Geometry check sheet. Reference: the model listing, model coordinates, mm. A direction names the side the tool comes from. Round coordinates to 2 decimals unless told otherwise and drop trailing zeros. Write each loop counter-clockwise with the first axis right and the second up, starting at its lowest first coordinate (ties: lowest second). Pieces come first, ordered by that corner, then holes. Notation, with made-up numbers: (18.5, 43) - (71.5, 43) arc R25 ccw to (71.5, 75) - close; hole circle Ø6 at (80.5, -34.5). An arc over 180 degrees is marked (long way). Return JSON: item names as keys, results as strings. Group by question number.
from build123d import *

# Parameters (mm, degrees)
SKETCH1_R               = 140
BOSS_EXTRUDE1_DEPTH     = 4
CUT_EXTRUDE1_REACH      = 6
CUT_EXTRUDE3_REACH      = 6
SKETCH19_R              = 1.5
CUT_EXTRUDE4_REACH      = 6
FILLET2_R               = 10
CUT_EXTRUDE8_DEPTH      = 1
CUT_EXTRUDE8_DEPTH_BACK = 5
CUT_EXTRUDE9_REACH      = 6
FILLET4_R               = 5
FILLET6_R               = 10
CUT_EXTRUDE10_REACH     = 6
SKETCH25_R              = 1.5
FILLET5_R               = 3


with BuildPart() as part:
    # Sketch1 → Boss-Extrude1 (new body)
    with BuildSketch(Plane(origin=(0, 0, 0), x_dir=(1, 0, 0), z_dir=(0, 1, 0))):
        Circle(SKETCH1_R)
    extrude(amount=BOSS_EXTRUDE1_DEPTH)

    # Sketch17 → Cut-Extrude1 (cut, up to next)
    with BuildSketch(Plane.XZ, mode=Mode.PRIVATE) as cut_extrude1_sk1:
        Polygon((-50, 90), (-121.24355653, 70), (-121.24355653, 140), (121.24355653, 140), (121.24355653, 70), (50, 90), align=None)
    cut_extrude1_tool1 = extrude(cut_extrude1_sk1.sketch, amount=-CUT_EXTRUDE1_REACH, mode=Mode.PRIVATE) & part.part
    add(cut_extrude1_tool1.solids().sort_by_distance((0, 0, 111.669853))[0], mode=Mode.SUBTRACT)

    # Sketch19 → Cut-Extrude3 (cut, up to next)
    with BuildSketch(Plane(origin=(0, 4, 0), x_dir=(1, 0, 0), z_dir=(0, 1, 0)), mode=Mode.PRIVATE) as cut_extrude3_sk1:
        with Locations((-79.195959493, -57.982756057)):
            Circle(SKETCH19_R)
    cut_extrude3_tool1 = extrude(cut_extrude3_sk1.sketch, amount=-CUT_EXTRUDE3_REACH, mode=Mode.PRIVATE) & part.part
    add(cut_extrude3_tool1.solids().sort_by_distance((-79.195959, 4, 57.982756))[0], mode=Mode.SUBTRACT)
    # Sketch19 → Cut-Extrude3 (cut, up to next)
    with BuildSketch(Plane(origin=(0, 4, 0), x_dir=(1, 0, 0), z_dir=(0, 1, 0)), mode=Mode.PRIVATE) as cut_extrude3_sk2:
        with Locations((-79.195959493, 57.982756057)):
            Circle(SKETCH19_R)
    cut_extrude3_tool2 = extrude(cut_extrude3_sk2.sketch, amount=-CUT_EXTRUDE3_REACH, mode=Mode.PRIVATE) & part.part
    add(cut_extrude3_tool2.solids().sort_by_distance((-79.195959, 4, -57.982756))[0], mode=Mode.SUBTRACT)
    # Sketch19 → Cut-Extrude3 (cut, up to next)
    with BuildSketch(Plane(origin=(0, 4, 0), x_dir=(1, 0, 0), z_dir=(0, 1, 0)), mode=Mode.PRIVATE) as cut_extrude3_sk3:
        with Locations((79.195959493, 57.982756057)):
            Circle(SKETCH19_R)
    cut_extrude3_tool3 = extrude(cut_extrude3_sk3.sketch, amount=-CUT_EXTRUDE3_REACH, mode=Mode.PRIVATE) & part.part
    add(cut_extrude3_tool3.solids().sort_by_distance((79.195959, 4, -57.982756))[0], mode=Mode.SUBTRACT)
    # Sketch19 → Cut-Extrude3 (cut, up to next)
    with BuildSketch(Plane(origin=(0, 4, 0), x_dir=(1, 0, 0), z_dir=(0, 1, 0)), mode=Mode.PRIVATE) as cut_extrude3_sk4:
        with Locations((79.195959493, -57.982756057)):
            Circle(SKETCH19_R)
    cut_extrude3_tool4 = extrude(cut_extrude3_sk4.sketch, amount=-CUT_EXTRUDE3_REACH, mode=Mode.PRIVATE) & part.part
    add(cut_extrude3_tool4.solids().sort_by_distance((79.195959, 4, 57.982756))[0], mode=Mode.SUBTRACT)
    # Sketch19 → Cut-Extrude3 (cut, up to next)
    with BuildSketch(Plane(origin=(0, 4, 0), x_dir=(1, 0, 0), z_dir=(0, 1, 0)), mode=Mode.PRIVATE) as cut_extrude3_sk5:
        with Locations((-57.982756057, 79.195959493)):
            Circle(SKETCH19_R)
    cut_extrude3_tool5 = extrude(cut_extrude3_sk5.sketch, amount=-CUT_EXTRUDE3_REACH, mode=Mode.PRIVATE) & part.part
    add(cut_extrude3_tool5.solids().sort_by_distance((-57.982756, 4, -79.195959))[0], mode=Mode.SUBTRACT)
    # Sketch19 → Cut-Extrude3 (cut, up to next)
    with BuildSketch(Plane(origin=(0, 4, 0), x_dir=(1, 0, 0), z_dir=(0, 1, 0)), mode=Mode.PRIVATE) as cut_extrude3_sk6:
        with Locations((57.982756057, 79.195959493)):
            Circle(SKETCH19_R)
    cut_extrude3_tool6 = extrude(cut_extrude3_sk6.sketch, amount=-CUT_EXTRUDE3_REACH, mode=Mode.PRIVATE) & part.part
    add(cut_extrude3_tool6.solids().sort_by_distance((57.982756, 4, -79.195959))[0], mode=Mode.SUBTRACT)
    # Sketch19 → Cut-Extrude3 (cut, up to next)
    with BuildSketch(Plane(origin=(0, 4, 0), x_dir=(1, 0, 0), z_dir=(0, 1, 0)), mode=Mode.PRIVATE) as cut_extrude3_sk7:
        with Locations((57.982756057, -79.195959493)):
            Circle(SKETCH19_R)
    cut_extrude3_tool7 = extrude(cut_extrude3_sk7.sketch, amount=-CUT_EXTRUDE3_REACH, mode=Mode.PRIVATE) & part.part
    add(cut_extrude3_tool7.solids().sort_by_distance((57.982756, 4, 79.195959))[0], mode=Mode.SUBTRACT)
    # Sketch19 → Cut-Extrude3 (cut, up to next)
    with BuildSketch(Plane(origin=(0, 4, 0), x_dir=(1, 0, 0), z_dir=(0, 1, 0)), mode=Mode.PRIVATE) as cut_extrude3_sk8:
        with Locations((-57.982756057, -79.195959493)):
            Circle(SKETCH19_R)
    cut_extrude3_tool8 = extrude(cut_extrude3_sk8.sketch, amount=-CUT_EXTRUDE3_REACH, mode=Mode.PRIVATE) & part.part
    add(cut_extrude3_tool8.solids().sort_by_distance((-57.982756, 4, 79.195959))[0], mode=Mode.SUBTRACT)

    # Sketch20 → Cut-Extrude4 (cut, up to next)
    with BuildSketch(Plane(origin=(0, 4, 0), x_dir=(1, 0, 0), z_dir=(0, 1, 0)), mode=Mode.PRIVATE) as cut_extrude4_sk1:
        Polygon((-498.316459894, 549.560016424), (-70, 121.24355653), (-50, 101.24355653), (50, 101.24355653), (70, 121.24355653), (498.316459894, 549.560016424), (498.316459894, 1761.021909565), (-498.316459894, 1761.021909565), align=None)
    cut_extrude4_tool1 = extrude(cut_extrude4_sk1.sketch, amount=-CUT_EXTRUDE4_REACH, mode=Mode.PRIVATE) & part.part
    add(cut_extrude4_tool1.solids().sort_by_distance((0, 4, -1025.243605))[0], mode=Mode.SUBTRACT)

    # Fillet2
    fillet2_edges = [part.edges().sort_by_distance(p)[0] for p in [
        (50, 2, -101.24355653),
        (-50, 2, -101.24355653),
    ]]
    fillet(fillet2_edges, radius=FILLET2_R)

    # Sketch23 → Cut-Extrude8 (cut, two sides)
    with BuildSketch(Plane(origin=(0, 4, 0), x_dir=(1, 0, 0), z_dir=(0, 1, 0))) as cut_extrude8_sk:
        with BuildLine():
            Line((261.924008605, 637.436261059), (-52.928932188, 104.172488718))
            ThreePointArc((-52.928932188, 104.172488718), (-80.130232259, 17.669229552), (-66.336519501, -71.95475195))
            Line((-66.336519501, -71.95475195), (-73.189737717, -96.367133919))
            Line((-73.189737717, -96.367133919), (-240.56703475, -692.594830068))
            Line((-240.56703475, -692.594830068), (918.053550165, -1130.326301498))
            Line((918.053550165, -1130.326301498), (1420.54459352, 199.704789628))
            Line((1420.54459352, 199.704789628), (261.924008605, 637.436261059))
        make_face()
    extrude(amount=CUT_EXTRUDE8_DEPTH, mode=Mode.SUBTRACT)
    extrude(cut_extrude8_sk.sketch, amount=-CUT_EXTRUDE8_DEPTH_BACK, mode=Mode.SUBTRACT)

    # Sketch24 → Cut-Extrude9 (cut, up to next)
    with BuildSketch(Plane(origin=(0, 4, 0), x_dir=(1, 0, 0), z_dir=(0, 1, 0)), mode=Mode.PRIVATE) as cut_extrude9_sk1:
        with BuildLine():
            Line((0, 0), (-100.308962252, 65.864346136))
            ThreePointArc((-100.308962252, 65.864346136), (-120, 0), (-100.308962252, -65.864346136))
            Line((-100.308962252, -65.864346136), (0, 0))
        make_face()
    cut_extrude9_tool1 = extrude(cut_extrude9_sk1.sketch, amount=-CUT_EXTRUDE9_REACH, mode=Mode.PRIVATE) & part.part
    add(cut_extrude9_tool1.solids().sort_by_distance((-75.574375, 4, 0))[0], mode=Mode.SUBTRACT)

    # Fillet4
    fillet4_edges = [part.edges().sort_by_distance(p)[0] for p in [
        (-74.063830686, 2, 48.63140512),
        (-75.142204111, 2, -49.339481038),
    ]]
    fillet(fillet4_edges, radius=FILLET4_R)

    # Fillet6
    fillet6_edges = [part.edges().sort_by_distance(p)[0] for p in [
        (-100.308962252, 2, 65.864346136),
        (-100.308962252, 2, -65.864346136),
    ]]
    fillet(fillet6_edges, radius=FILLET6_R)

    # Sketch25 → Cut-Extrude10 (cut, up to next)
    with BuildSketch(Plane(origin=(0, 4, 0), x_dir=(1, 0, 0), z_dir=(0, 1, 0)), mode=Mode.PRIVATE) as cut_extrude10_sk1:
        with Locations((-120, 50)):
            Circle(SKETCH25_R)
    cut_extrude10_tool1 = extrude(cut_extrude10_sk1.sketch, amount=-CUT_EXTRUDE10_REACH, mode=Mode.PRIVATE) & part.part
    add(cut_extrude10_tool1.solids().sort_by_distance((-120, 4, -50))[0], mode=Mode.SUBTRACT)
    # Sketch25 → Cut-Extrude10 (cut, up to next)
    with BuildSketch(Plane(origin=(0, 4, 0), x_dir=(1, 0, 0), z_dir=(0, 1, 0)), mode=Mode.PRIVATE) as cut_extrude10_sk2:
        with Locations((-120, -50)):
            Circle(SKETCH25_R)
    cut_extrude10_tool2 = extrude(cut_extrude10_sk2.sketch, amount=-CUT_EXTRUDE10_REACH, mode=Mode.PRIVATE) & part.part
    add(cut_extrude10_tool2.solids().sort_by_distance((-120, 4, 50))[0], mode=Mode.SUBTRACT)

    # Fillet5
    fillet5_edges = [part.edges().sort_by_distance(p)[0] for p in [
        (-121.24355653, 2, 70),
        (-70, 2, -121.24355653),
        (-52.928932188, 2, -104.172488718),
        (-69.838855295, 2, 84.430694855),
        (-66.336519501, 2, 71.95475195),
    ]]
    fillet(fillet5_edges, radius=FILLET5_R)


solid = part.part
1. Section check B-B (z = 66). Enter the section's corners in (x, y).
2. Tool access check on faces 4 (the face through (-69.68, 2.03, 63.01)), 5 (the face through (-70.476, 1.972, 83.363)), 6 (the face through (-86.2, 2, -56.6)). Record the directions out of +Z, -Z, +X, -X, +Y, -Y that give a thin tool (end or side, any length) a straight path to the whole face; none if there is none.
3. Depth check by flat-ended pin: pin 1 Ø4 at (x, z) = (-79.2, -57.98) entering from +Y; pin 2 Ø2 at (y, z) = (1, 34.5) entering from -X; pin 3 Ø1.8 at (x, z) = (-120, -50) entering from +Y; pin 4 Ø1 at (y, z) = (2.5, -43) entering from +X. Enter the tip coordinate at first touch or a pass-through.
4. Section check A-A (y = 2.1). Enter the section's corners in (x, z) (3 decimals).
5. Material ranges on line 1 along X through (y, z) = (0.9, 50); line 2 along Z through (x, y) = (-75, 2.7); line 3 along X through (y, z) = (1.2, 1), recorded low to high.
6. Mould release check, pull along X, two halves, no side actions. Record for faces 1 (the face through (-67.803, 2.028, 77.177)), 2 (the face through (-123, 4, -26)), 3 (the face through (-75.373, 2.028, 51.834)): pulls with the +X half, pulls with the -X half, needs draft (parallel to the pull), parting line crosses it, or undercut.
Result sheet:
{
 "1": {"outline": "(-123.47, 0) - (-68.62, 0) - (-68.62, 4) - (-123.47, 4) - close"},
 "2": {"face 4": "+X, +Y, -Y", "face 5": "+Z, +Y, -Y", "face 6": "+Y, -Y"},
 "3": {"pin 1": "stops at y = 4", "pin 2": "stops at x = -135.93", "pin 3": "passes through", "pin 4": "stops at x = -111.84"},
 "4": {"outline": "(-121.86, 68.921) arc R140 ccw to (-72.023, -120.053) arc R3 ccw to (-68.358, -119.602) - (-54.563, -105.807) arc R3 ccw to (-54.084, -102.19) arc R200 cw to (-73.413, -56.011) arc R5 ccw to (-80.975, -53.169) - (-91.569, -60.126) arc R10 cw to (-105.881, -56.473) arc R120 cw to (-105.881, 56.473) arc R10 cw to (-91.569, 60.126) - (-79.765, 52.375) arc R5 ccw to (-72.233, 55.114) arc R200 cw to (-66.709, 71.019) arc R3 ccw to (-66.611, 72.932) - (-69.028, 81.542) arc R3 ccw to (-72.727, 83.62) - (-120.06, 70.332) arc R3 ccw to start; hole circle Ø3 at (-120, -50); hole circle Ø3 at (-120, 50); hole circle Ø3 at (-79.196, -57.983); hole circle Ø3 at (-79.196, 57.983)"},
 "5": {"line 1": "x = -130.77 to -121.5, -118.5 to -109.09", "line 2": "z = -118.22 to -53.53, 51.98 to 82.98", "line 3": "x = -140 to -120"},
 "6": {"face 1": "pulls with the +X half", "face 2": "needs draft", "face 3": "undercut"}
}
